from build123d import *

# Parameters (mm, degrees)
SKETCH1_W           = 25
SKETCH1_H           = 30
BOSS_EXTRUDE1_DEPTH = 30
SKETCH3_W           = 3
SKETCH3_H           = 3
CUT_EXTRUDE1_DEPTH  = 16
CUT_EXTRUDE2_DEPTH  = 4.8
FILLET1_R           = 10
FILLET2_R           = 3


# Some blends are built 0.0001 mm under size
with BuildPart() as part:
    # Sketch1 → Boss-Extrude1 (new body)
    with BuildSketch(Plane(origin=(0, 0, 0), x_dir=(1, 0, 0), z_dir=(0, 1, 0))):
        Rectangle(SKETCH1_W, SKETCH1_H)
    extrude(amount=BOSS_EXTRUDE1_DEPTH)

    # Sketch3 → Cut-Extrude1 (cut)
    with BuildSketch(Plane(origin=(12.5, 0, 0), x_dir=(0, 0, -1), z_dir=(1, 0, 0))):
        with Locations((10.5, 25.5)):
            Rectangle(SKETCH3_W, SKETCH3_H)
        with Locations((-10.5, 25.5)):
            Rectangle(SKETCH3_W, SKETCH3_H)
    extrude(amount=-CUT_EXTRUDE1_DEPTH, mode=Mode.SUBTRACT)

    # Sketch5 → Cut-Extrude2 (cut)
    with BuildSketch(Plane(origin=(0, 30, 0), x_dir=(1, 0, 0), z_dir=(0, 1, 0))):
        with BuildLine():
            Line((-12.5, -12), (-1.5, -12))
            Line((-1.5, -12), (-1.5, -8.5))
            ThreePointArc((-1.5, -8.5), (7, 0), (-1.5, 8.5))
            Line((-1.5, 8.5), (-1.5, 12))
            Line((-1.5, 12), (-12.5, 12))
            Line((-12.5, 12), (-12.5, -12))
        make_face()
    extrude(amount=-CUT_EXTRUDE2_DEPTH, mode=Mode.SUBTRACT)

    # Fillet1
    # the kernel refuses this fillet: 10 mm, written as the material it takes off along each edge
    with BuildSketch(Plane(origin=(-1.5, 40.838231957, 8.5), x_dir=(0, 0, 1), z_dir=(0, -1, 0))) as fillet1_piece_1:
        with BuildLine():
            CenterArc((7.59375, -9.123662145), FILLET1_R, 114.165579325, 36.285209338)
            Line((-1.105574324, -4.191952877), (-1.279560811, -4.093318692))
            ThreePointArc((-1.279560811, -4.093318692), (-0.474426959, -2.116642947), (-0.2, 0))
            Line((-0.2, 0), (0, 0.2))
            ThreePointArc((0, 0.2), (1.75, 0.2), (3.418125, 0.182473243))
            Line((3.418125, 0.182473243), (3.5, 0))
        make_face()
    extrude(amount=15.638231957, mode=Mode.SUBTRACT)
    with BuildSketch(Plane(origin=(-1.5, 40.838231957, -8.5), x_dir=(0.9669365109541641, 0, 0.2550172225238677), z_dir=(0, -1, 0))) as fillet1_piece_2:
        with BuildLine():
            CenterArc((6.885465008, -9.66936511), FILLET1_R, 104.774605668, 36.285209338)
            Line((-0.892560279, -3.384277788), (-1.048120785, -3.258576042))
            ThreePointArc((-1.048120785, -3.258576042), (-0.639667442, -1.64113545), (-0.193387302, 0.051003445))
            Line((-0.193387302, 0.051003445), (0.051003445, 0.193387302))
            ThreePointArc((0.051003445, 0.193387302), (2.167646391, -0.081039657), (4.284289338, 0.193387302))
            Line((4.284289338, 0.193387302), (4.335292783, 0))
        make_face()
    extrude(amount=15.638231957, mode=Mode.SUBTRACT)

    # Fillet2
    fillet2_edges = [part.edges().sort_by_distance(p)[0] for p in [
        (-12.5, 27.6, 12),
        (-12.5, 27.6, -12),
    ]]
    fillet(fillet2_edges, radius=FILLET2_R - 0.0001)  # a hair under: the kernel refuses the full size


solid = part.part
For this review, take the finished solid that the model builds, in its own axes (mm). A direction names the side the tool comes from. Coordinates: 2 decimals unless noted, no trailing zeros. Order: outer loops, then holes, each group sorted by start corner. A loop starts at its lowest first (then second) coordinate and runs counter-clockwise, first axis right, second up. Notation, with made-up numbers: (1.25, 69.25) - (21.25, 69.25) arc R27 cw to (21.25, 105.25) - close; hole circle Ø5 at (27.5, -0.75). An arc over 180 degrees is marked (long way). Answer as CSV lines item,"result". Start each with the question number.
1) Add section D-D (z = 3.25). State the section outline as (x, y) points.
2) Draft analysis for pull direction Z (two halves, no side actions). For faces 5 (the flat face through (12.5, 15, 0)), 6 (the cylindrical face through (7, 28, 0)), 7 (the flat face through (0, 15, 15)), state which applies: +Z half, -Z half, draft (parallel to the pull), parting line (faces both ways), or undercut.
3) Machinability: for faces 1 (the flat face through (5, 25, 9)), 2 (the cylindrical face through (0.199, 28.167, 9.395)), 3 (the flat face through (-3.5, 25, -10)), 4 (the flat face through (-1, 26, -12)), which of the approach directions +Z, -Z, +X, -X, +Y, -Y give a long, thin tool a straight path to every point of the face, cutting with its end or side? Answer none if there is none.
4) Add section C-C (x = -8.75). State the section outline as (y, z) points.
5) Add section A-A (y = 24.5). State the section outline as (x, z) points.
6) Add section B-B (x = 7.5). State the section outline as (y, z) points.
7) To check wall thickness, follow line 1 along Z through (x, y) = (-6, 26.75); line 2 along Y through (x, z) = (8.75, 11.25); line 3 along Y through (x, z) = (-9.25, -0.5). State the ranges of each line that lie inside material, in increasing order. Write a range as [from, to].
8) Insertion check: P1, Ø6, axis at x = -6, z = -8.5, coming from the +Y side; P2, Ø1, axis at y = 25, z = 10.5, coming from the +X side. Each pin has a flat end and moves straight along its axis. Give the tip position at first contact, or say it passes through.
Result:
1,outline,"(-12.5, 0) - (12.5, 0) - (12.5, 30) - (6.35, 30) - (6.35, 25.2) - (-12.5, 25.2) - close"
2,face 5,"draft"
2,face 6,"undercut"
2,face 7,"+Z half"
3,face 1,"+X"
3,face 2,"-X, +Y"
3,face 3,"+X, +Y"
3,face 4,"none"
4,outline,"(0, -15) - (30, -15) - (30, -12) - (25.2, -12) - (25.2, 12) - (30, 12) - (30, 15) - (0, 15) - close"
5,outline,"(-12.5, -15) - (12.5, -15) - (12.5, -12) - (-3.5, -12) - (-3.5, -9) - (12.5, -9) - (12.5, 9) - (-3.5, 9) - (-3.5, 12) - (12.5, 12) - (12.5, 15) - (-12.5, 15) - close"
6,outline,"(0, -15) - (30, -15) - (30, 15) - (0, 15) - close; hole (24, -12) - (27, -12) - (27, -9) - (24, -9) - close; hole (24, 9) - (27, 9) - (27, 12) - (24, 12) - close"
7,line 1,"[-15, -12], [12, 15]"
7,line 2,"[0, 24], [27, 30]"
7,line 3,"[0, 25.2]"
8,P1,"y = 25.2"
8,P2,"x = -3.5"
